Model file for the job. Use its own axes, mm. A direction names the side the tool comes from. Round coordinates to 2 decimals unless told otherwise and drop trailing zeros. Write each loop counter-clockwise with the first axis right and the second up, starting at its lowest first coordinate (ties: lowest second). Pieces come first, ordered by that corner, then holes. Notation, with made-up numbers: (27.5, 78) - (39.5, 78) arc R11 cw to (39.5, 90) - close; hole circle Ø10 at (-4, -31.75). An arc over 180 degrees is marked (long way). One line per item, written item: value.
from build123d import *

# Parameters (mm, degrees)
F0_W          = 77.12
F0_H          = 39.56
F0_W_2        = 2
F0_H_2        = 6
F1_DEPTH      = 2
F2_DEPTH      = 8
F2_DEPTH_BACK = -2
F3_DEPTH      = 8
F3_DEPTH_BACK = -2
F4_W          = 6
F4_H          = 3
F5_DEPTH      = 4
F6_W          = 6
F6_H          = 3
F7_DEPTH      = 4


with BuildPart() as f1:
    # F0 (on Top) → F1 (new body)
    with BuildSketch(Plane.XY):
        with Locations((38.56, 19.78)):
            Rectangle(F0_W, F0_H)
        with Locations((4, 10.89)):
            Rectangle(F0_W_2, F0_H_2, mode=Mode.SUBTRACT)
        with BuildLine():
            ThreePointArc((15.892051, 23.32), (16.091852, 22.837638), (16.16, 22.32))
            ThreePointArc((16.16, 22.32), (13.642362, 20.388148), (12.427949, 23.32))
            Line((12.427949, 23.32), (8.831288, 23.32))
            ThreePointArc((8.831288, 23.32), (8.987266, 22.830774), (9.04, 22.32))
            ThreePointArc((9.04, 22.32), (6.029226, 19.872734), (4.248712, 23.32))
            Line((4.248712, 23.32), (2.73, 23.32))
            Line((2.73, 23.32), (2.73, 25.32))
            Line((2.73, 25.32), (71.31, 25.32))
            Line((71.31, 25.32), (71.31, 23.32))
            Line((71.31, 23.32), (69.791288, 23.32))
            ThreePointArc((69.791288, 23.32), (69.947266, 22.830774), (70, 22.32))
            ThreePointArc((70, 22.32), (66.989226, 19.872734), (65.208712, 23.32))
            Line((65.208712, 23.32), (61.612051, 23.32))
            ThreePointArc((61.612051, 23.32), (61.811852, 22.837638), (61.88, 22.32))
            ThreePointArc((61.88, 22.32), (59.362362, 20.388148), (58.147949, 23.32))
            Line((58.147949, 23.32), (53.992051, 23.32))
            ThreePointArc((53.992051, 23.32), (54.191852, 22.837638), (54.26, 22.32))
            ThreePointArc((54.26, 22.32), (51.742362, 20.388148), (50.527949, 23.32))
            Line((50.527949, 23.32), (46.372051, 23.32))
            ThreePointArc((46.372051, 23.32), (46.571852, 22.837638), (46.64, 22.32))
            ThreePointArc((46.64, 22.32), (44.122362, 20.388148), (42.907949, 23.32))
            Line((42.907949, 23.32), (38.752051, 23.32))
            ThreePointArc((38.752051, 23.32), (38.951852, 22.837638), (39.02, 22.32))
            ThreePointArc((39.02, 22.32), (36.502362, 20.388148), (35.287949, 23.32))
            Line((35.287949, 23.32), (31.132051, 23.32))
            ThreePointArc((31.132051, 23.32), (31.331852, 22.837638), (31.4, 22.32))
            ThreePointArc((31.4, 22.32), (28.882362, 20.388148), (27.667949, 23.32))
            Line((27.667949, 23.32), (23.512051, 23.32))
            ThreePointArc((23.512051, 23.32), (23.711852, 22.837638), (23.78, 22.32))
            ThreePointArc((23.78, 22.32), (21.262362, 20.388148), (20.047949, 23.32))
            Line((20.047949, 23.32), (15.892051, 23.32))
        make_face(mode=Mode.SUBTRACT)
        with Locations((73.12, 28.67)):
            Rectangle(F0_W_2, F0_H_2, mode=Mode.SUBTRACT)
        with BuildLine():
            ThreePointArc((12.082051, 36.02), (12.281852, 35.537638), (12.35, 35.02))
            ThreePointArc((12.35, 35.02), (9.832362, 33.088148), (8.617949, 36.02))
            Line((8.617949, 36.02), (6.54, 36.02))
            Line((6.54, 36.02), (6.54, 38.02))
            Line((6.54, 38.02), (75.12, 38.02))
            Line((75.12, 38.02), (75.12, 36.02))
            Line((75.12, 36.02), (73.042051, 36.02))
            ThreePointArc((73.042051, 36.02), (73.241852, 35.537638), (73.31, 35.02))
            ThreePointArc((73.31, 35.02), (70.792362, 33.088148), (69.577949, 36.02))
            Line((69.577949, 36.02), (65.422051, 36.02))
            ThreePointArc((65.422051, 36.02), (65.621852, 35.537638), (65.69, 35.02))
            ThreePointArc((65.69, 35.02), (63.172362, 33.088148), (61.957949, 36.02))
            Line((61.957949, 36.02), (57.802051, 36.02))
            ThreePointArc((57.802051, 36.02), (58.001852, 35.537638), (58.07, 35.02))
            ThreePointArc((58.07, 35.02), (55.552362, 33.088148), (54.337949, 36.02))
            Line((54.337949, 36.02), (50.182051, 36.02))
            ThreePointArc((50.182051, 36.02), (50.381852, 35.537638), (50.45, 35.02))
            ThreePointArc((50.45, 35.02), (47.932362, 33.088148), (46.717949, 36.02))
            Line((46.717949, 36.02), (42.562051, 36.02))
            ThreePointArc((42.562051, 36.02), (42.761852, 35.537638), (42.83, 35.02))
            ThreePointArc((42.83, 35.02), (40.312362, 33.088148), (39.097949, 36.02))
            Line((39.097949, 36.02), (34.942051, 36.02))
            ThreePointArc((34.942051, 36.02), (35.141852, 35.537638), (35.21, 35.02))
            ThreePointArc((35.21, 35.02), (32.692362, 33.088148), (31.477949, 36.02))
            Line((31.477949, 36.02), (27.322051, 36.02))
            ThreePointArc((27.322051, 36.02), (27.521852, 35.537638), (27.59, 35.02))
            ThreePointArc((27.59, 35.02), (25.072362, 33.088148), (23.857949, 36.02))
            Line((23.857949, 36.02), (19.702051, 36.02))
            ThreePointArc((19.702051, 36.02), (19.901852, 35.537638), (19.97, 35.02))
            ThreePointArc((19.97, 35.02), (17.452362, 33.088148), (16.237949, 36.02))
            Line((16.237949, 36.02), (12.082051, 36.02))
        make_face(mode=Mode.SUBTRACT)
    extrude(amount=F1_DEPTH)

    # F0 (on Top) → F2 (join, two sides)
    with BuildSketch(Plane.XY) as f2_sk:
        with Locations((73.12, 28.67)):
            Rectangle(F0_W_2, F0_H_2)
    extrude(amount=-F2_DEPTH)
    extrude(f2_sk.sketch, amount=-F2_DEPTH_BACK)

    # F0 (on Top) → F3 (join, two sides)
    with BuildSketch(Plane.XY) as f3_sk:
        with Locations((4, 10.89)):
            Rectangle(F0_W_2, F0_H_2)
    extrude(amount=-F3_DEPTH)
    extrude(f3_sk.sketch, amount=-F3_DEPTH_BACK)

    # F4 (on face) → F5 (join)
    with BuildSketch(Plane.YZ.offset(5)):
        with Locations((10.89, -6.5)):
            Rectangle(F4_W, F4_H)
    extrude(amount=-F5_DEPTH)

    # F6 (on face) → F7 (join)
    with BuildSketch(Plane(origin=(72.12, 0, 0), x_dir=(0, -1, 0), z_dir=(-1, 0, 0))):
        with Locations((-28.67, -6.5)):
            Rectangle(F6_W, F6_H)
    extrude(amount=-F7_DEPTH)


solid = f1.part
1. Band-saw the part on B-B on z = -6.5. Write the cut outline in (x, y).
Report:
outline: (1, 7.89) - (5, 7.89) - (5, 13.89) - (1, 13.89) - close; (72.12, 25.67) - (76.12, 25.67) - (76.12, 31.67) - (72.12, 31.67) - close
2. Band-saw the part on D-D on z = -3. Write the cut outline in (x, y), plus the area to 3 significant figures.
Report:
outline: (3, 7.89) - (5, 7.89) - (5, 13.89) - (3, 13.89) - close; (72.12, 25.67) - (74.12, 25.67) - (74.12, 31.67) - (72.12, 31.67) - close
area: 24.0 mm²
3. Drop flat-ended pins along their axis: pin 1 (3 mm diameter, centred on x = 2.5, z = -6, fed in from -Y); pin 2 (10 mm diameter, centred on x = 47, y = 8, fed in from -Z); pin 3 (2 mm diameter, centred on y = 12.5, z = -1.5, fed in from +X); pin 4 (2.5 mm diameter, centred on x = 29.4, y = 22.32, fed in from +Z). Give the stop position or say it passes through.
Report:
pin 1: y = 7.89
pin 2: z = 0
pin 3: x = 5
pin 4: through
4. Band-saw the part on C-C on x = 67.5. Write the cut outline in (y, z), plus the area to 3 significant figures.
Report:
outline: (0, 0) - (19.82, 0) - (19.82, 2) - (0, 2) - close; (25.32, 0) - (36.02, 0) - (36.02, 2) - (25.32, 2) - close; (38.02, 0) - (39.56, 0) - (39.56, 2) - (38.02, 2) - close
area: 64.1 mm²
5. Mould opens along X. For faces 1 (the face through (3, 11, -2)), 2 (the face through (40, 38.02, 1)), 3 (the face through (38, 16, 0)) say: released by +X, released by -X, zero draft, split by the parting line, or undercut.
Report:
face 1: released by -X
face 2: undercut
face 3: zero draft
6. Tool access for faces 4 (the face through (73.6, 31.67, -4.8)), 5 (the face through (18, 23.32, 1)), 6 (the face through (73.6, 25.67, -4.8)), 7 (the face through (3, 11, -8)), 8 (the face through (77.12, 20, 1)): list every direction of +Z, -Z, +X, -X, +Y, -Y with a clear straight run to the whole face (end or side of a thin tool).
Report:
face 4: -Z, +X, -X, +Y
face 5: +Z, -Z
face 6: -Z, +X, -X, -Y
face 7: -Z, +X, -X, +Y, -Y
face 8: +Z, -Z, +X, +Y, -Y
7. Band-saw the part on A-A on x = 29.4. Write the cut outline in (y, z).
Report:
outline: (0, 0) - (20.32, 0) - (20.32, 2) - (0, 2) - close; (25.32, 0) - (36.02, 0) - (36.02, 2) - (25.32, 2) - close; (38.02, 0) - (39.56, 0) - (39.56, 2) - (38.02, 2) - close
8. Wall check: probe 1 along Y at (x, z) = (25.59, 1.45); probe 2 along Y at (x, z) = (37.02, 1.2); probe 3 along Z at (x, y) = (47, 3). Give the ranges that are in metal, low to high. Write a range as [from, to].
Report:
probe 1: [0, 23.32], [25.32, 33.02], [38.02, 39.56]
probe 2: [0, 20.32], [25.32, 36.02], [38.02, 39.56]
probe 3: [0, 2]
